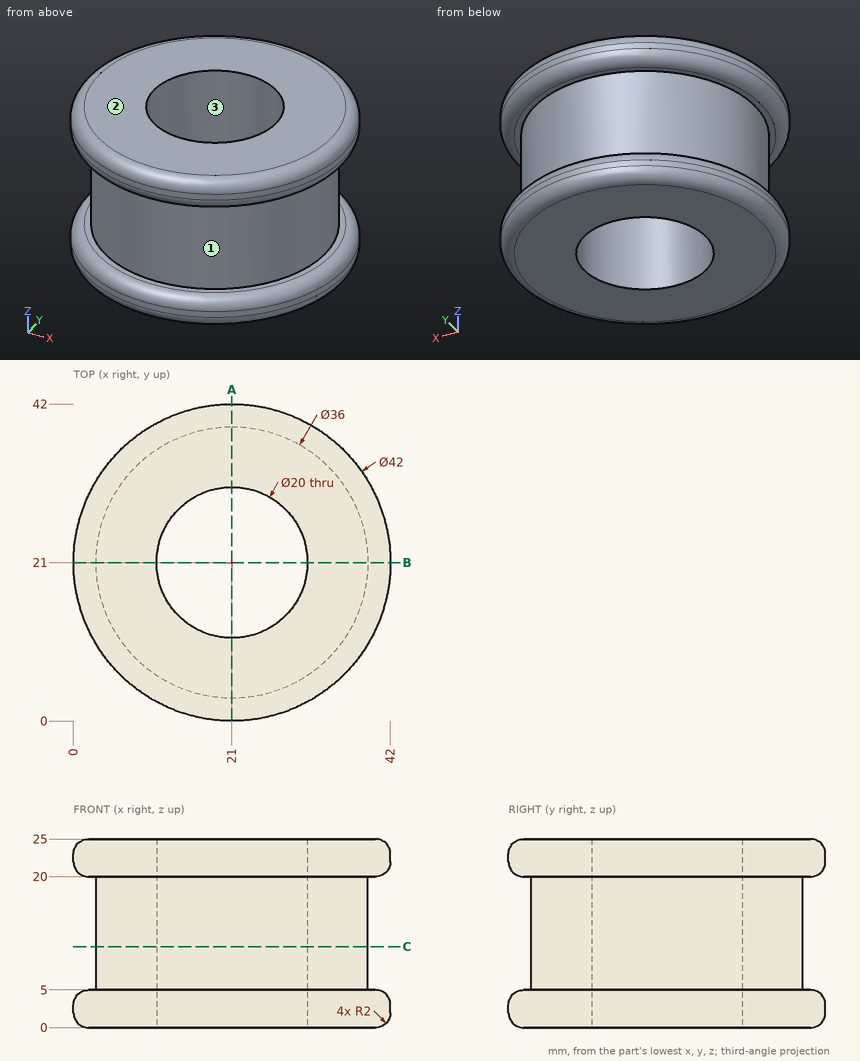
Verification items for this drawing (mm, ordinates from the low corner). Coordinates: 2 decimals unless noted, no trailing zeros. Loops run counter-clockwise (first coordinate to the right, second up) from the corner with the lowest first, then second, coordinate; pieces in that order, holes last. Notation, with made-up numbers: (51.25, 82) - (97.25, 82) arc R27 ccw to (97.25, 98) - close; hole circle Ø5 at (-24.5, 52). An arc over 180 degrees is marked (long way). Use one line per item in the form item = value. Start each with the question number.
Item 1: Section check A-A, the plane x = 21. Enter the section's corners in (y, z), and give its area (3 significant figures).
Item 2: Mould release check, pull along X, two halves, no side actions. Record for the marked faces 1, 2 and 3: +X half, -X half, draft (parallel to the pull), parting line (faces both ways), or undercut.
Item 3: Thickness scan on probe 1 along X at (y, z) = (21, 6.5); probe 2 along Y at (x, z) = (20.5, 11); probe 3 along Z at (x, y) = (36.5, 35). Record the ranges inside material, lowest first.
Item 4: Gauge pin test, flat ends, axial feed: pin 1 (2 mm diameter, centred on x = 31.5, z = 18.5, fed in from -Y); pin 2 (5 mm diameter, centred on y = 16.5, z = 4, fed in from -X); pin 3 (5 mm diameter, centred on y = 29.5, z = 7, fed in from +X); pin 4 (12 mm diameter, centred on x = 21, y = 21, fed in from +Z). Record the tip position at first contact, or that the pin passes through.
Item 5: Section check C-C, the plane z = 10.75. Enter the section's corners in (x, y), and give its area (3 significant figures).
Computed:
q1.outline = (0, 2) arc R2 ccw to (2, 0) - (11, 0) - (11, 25) - (2, 25) arc R2 ccw to (0, 23) - (0, 22) arc R2 ccw to (2, 20) - (3, 20) - (3, 5) - (2, 5) arc R2 ccw to (0, 3) - close; (31, 0) - (40, 0) arc R2 ccw to (42, 2) - (42, 3) arc R2 ccw to (40, 5) - (39, 5) - (39, 20) - (40, 20) arc R2 ccw to (42, 22) - (42, 23) arc R2 ccw to (40, 25) - (31, 25) - close
q1.area = 453 mm2
q2.face_1 = parting line
q2.face_2 = draft
q2.face_3 = undercut
q3.probe_1 = 3 to 11, 31 to 39
q3.probe_2 = 3.01 to 11.01, 30.99 to 38.99
q3.probe_3 = 1.34 to 3.66, 21.34 to 23.66
q4.pin_1 = 5.71
q4.pin_2 = 0.11
q4.pin_3 = 39.63
q4.pin_4 = through
q5.outline = circle Ø36 at (21, 21); hole circle Ø20 at (21, 21)
q5.area = 704 mm2
